Build history of the part. All positions in model axes, mm. A direction names the side the tool comes from. Round coordinates to 2 decimals unless told otherwise and drop trailing zeros. Order: outer loops, then holes, each group sorted by start corner. A loop starts at its lowest first (then second) coordinate and runs counter-clockwise, first axis right, second up. Notation, with made-up numbers: (-32, 6.5) -> (-20, 6.5) arc R25 cw to (-20, 26.5) -> close; hole circle Ø1 at (52.25, 52). An arc over 180 degrees is marked (long way). Use a Markdown table: item, result. Add a question column.
Item 1: Slice it at B-B, the plane x = -15. Give the cut face in (y, z).
Item 2: 3-axis set-ups, long thin cutter, end or side, ignore diameter. For faces 1 (the face through (4.93, -39.847, 20.421)), 2 (the face through (4.93, -4.292, 41.025)), 3 (the face through (4.93, 28.062, 34.767)): which of +Z, -Z, +X, -X, +Y, -Y reach the whole face in a straight line?
Item 3: Slice it at C-C, the plane z = 27.5. Give the cut face in (x, y).
Item 4: Two-plate mould, pull along Y, no slides. Class faces 4 (the face through (4.93, -24.39, 37.43)), 5 (the face through (4.93, 39.78, 20.35)), 6 (the face through (4.93, -40.35, -8.56)): released by +Y, released by -Y, zero draft, split by the parting line, or undercut.
Item 5: Probe L1, parallel to Y at x = -5, z = 0; L2, parallel to Y at x = -12.5, z = -16.5; L3, parallel to X at y = 33, z = -4. List the from-to ranges inside material, lowest first.
Item 6: Slice it at D-D, the plane y = 23.5. Give the cut face in (x, z), plus the area to 3 significant figures.
Item 7: Slice it at A-A, the plane z = 0. Give the cut face in (x, y).
Item 8: Pin check, flat tips, straight feed: pin 1 (7.5 mm diameter, centred on x = -10.5, z = 4.5, fed in from -Y); pin 2 (5 mm diameter, centred on x = 2.5, y = 34, fed in from +Z); pin 3 (10 mm diameter, centred on x = -15.5, z = 17.5, fed in from +Y). Stop position of each tip, or through.
from build123d import *

# Parameters (mm, degrees)
BASPROSKE_W         = 10
BASPROSKE_H         = 48
TOOTHCUT_DEPTH      = 69.614867194
TEETHCUTS_COUNT     = 30
TEETHCUTS_ANGLE     = 348
BORSKE_R            = 5
BORE_DEPTH          = 50.0000508
SKETCH2_W           = 44.6
SKETCH2_H           = 44.6
BOSS_EXTRUDE1_DEPTH = 60
CUT_EXTRUDE1_REACH  = 99.421
SKETCH1_R           = 7.7
CUT_EXTRUDE2_REACH  = 106.024
SKETCH3_W           = 35
SKETCH3_H           = 44.6
FILLET1_R           = 2


with BuildPart() as part:
    # BasProSke → Base-Revolve (revolve)
    with BuildSketch(Plane(origin=(0, 0, 0), x_dir=(1, 0, 0), z_dir=(0, 1, 0)), mode=Mode.PRIVATE) as base_revolve_sk:
        with Locations((5, 24)):
            Rectangle(BASPROSKE_W, BASPROSKE_H)
    revolve(base_revolve_sk.sketch.rotate(Axis((-10, 0, 0), (1, 0, 0)), 180), axis=Axis((-10, 0, 0), (1, 0, 0)))

    # TooCutSke → ToothCut (cut, through all)
    with BuildSketch(Plane(origin=(0, 0, 0), x_dir=(0, 0, -1), z_dir=(1, 0, 0))):
        with BuildLine():
            ThreePointArc((1.388358102, 41.225628713), (0, 41.249), (-1.388358102, 41.225628713))
            ThreePointArc((-1.388358102, 41.225628713), (-2.434419088, 44.674608087), (-4.146627223, 47.846050285))
            ThreePointArc((-4.146627223, 47.846050285), (0, 48.0254), (4.146627223, 47.846050285))
            ThreePointArc((4.146627223, 47.846050285), (2.434419088, 44.674608087), (1.388358102, 41.225628713))
        make_face()
    toothcut = extrude(amount=TOOTHCUT_DEPTH, mode=Mode.SUBTRACT)

    # TeethCuts: ToothCut ×30 about axis
    teethcuts_axis = Axis((-10, 0, 0), (1, 0, 0))
    for i in range(1, TEETHCUTS_COUNT):
        add(toothcut.rotate(teethcuts_axis, i * TEETHCUTS_ANGLE / (TEETHCUTS_COUNT - 1)), mode=Mode.SUBTRACT)

    # BorSke → Bore (cut, symmetric)
    with BuildSketch(Plane(origin=(0, 0, 0), x_dir=(0, 0, -1), z_dir=(1, 0, 0))):
        with Locations(Location((0, 0, 0), (0, 0, 180))):
            Circle(BORSKE_R)
    extrude(amount=BORE_DEPTH, both=True, mode=Mode.SUBTRACT)

    # Sketch2 → Boss-Extrude1 (add)
    with BuildSketch(Plane.ZY):
        Rectangle(SKETCH2_W, SKETCH2_H)
    extrude(amount=BOSS_EXTRUDE1_DEPTH)

    # Sketch1 → Cut-Extrude1 (cut, up to next)
    with BuildSketch(Plane(origin=(10, 0, 0), x_dir=(0, 0, -1), z_dir=(1, 0, 0)), mode=Mode.PRIVATE) as cut_extrude1_sk1:
        Circle(SKETCH1_R)
    cut_extrude1_tool1 = extrude(cut_extrude1_sk1.sketch, amount=-CUT_EXTRUDE1_REACH, mode=Mode.PRIVATE) & part.part
    add(cut_extrude1_tool1.solids().sort_by_distance((10, 0, 0))[0], mode=Mode.SUBTRACT)

    # Sketch3 → Cut-Extrude2 (cut, up to next)
    with BuildSketch(Plane(origin=(0, 22.3, 0), x_dir=(1, 0, 0), z_dir=(0, 1, 0)), mode=Mode.PRIVATE) as cut_extrude2_sk1:
        with Locations((-42.5, 0)):
            Rectangle(SKETCH3_W, SKETCH3_H)
    cut_extrude2_tool1 = extrude(cut_extrude2_sk1.sketch, amount=-CUT_EXTRUDE2_REACH, mode=Mode.PRIVATE) & part.part
    add(cut_extrude2_tool1.solids().sort_by_distance((-42.5, 22.3, 0))[0], mode=Mode.SUBTRACT)

    # Fillet1
    fillet1_edges = [part.edges().sort_by_distance(p)[0] for p in [
        (10, 0, 7.7),
        (-25, 0, 7.7),
    ]]
    fillet(fillet1_edges, radius=FILLET1_R)


solid = part.part
Check sheet entries:
| question | item | result |
|---|---|---|
| 1 | outline | (-22.3, -22.3) -> (22.3, -22.3) -> (22.3, 22.3) -> (-22.3, 22.3) -> close; hole circle Ø15.4 at (0, 0) |
| 2 | face 1 | +X, -X, -Y |
| 2 | face 2 | +Z, +X, -X |
| 2 | face 3 | +X, -X |
| 3 | outline | (0, -34.24) -> (10, -34.24) -> (10, 34.24) -> (0, 34.24) -> close |
| 4 | face 4 | undercut |
| 4 | face 5 | released by +Y |
| 4 | face 6 | released by -Y |
| 5 | L1 | -22.3 to -7.7, 7.7 to 22.3 |
| 5 | L2 | -22.3 to 22.3 |
| 5 | L3 | 0 to 10 |
| 6 | outline | (0, -36.7) -> (10, -36.7) -> (10, 36.7) -> (0, 36.7) -> close |
| 6 | area | 734 mm2 |
| 7 | outline | (-25, -22.3) -> (0, -22.3) -> (0, -41.25) -> (10, -41.25) -> (10, -9.7) arc R2 ccw to (8, -7.7) -> (-23, -7.7) arc R2 ccw to (-25, -9.7) -> close; (-25, 9.7) arc R2 ccw to (-23, 7.7) -> (8, 7.7) arc R2 ccw to (10, 9.7) -> (10, 41.25) -> (0, 41.25) -> (0, 22.3) -> (-25, 22.3) -> close |
| 8 | pin 1 | y = -22.3 |
| 8 | pin 2 | z = 32.77 |
| 8 | pin 3 | y = 22.3 |
